```python
from build123d import *

# Parameters (mm, degrees)
F1_DEPTH = 12.7


with BuildPart() as f1:
    # F0 (on Front) → F1 (new body, symmetric)
    with BuildSketch(Plane.XZ):
        with BuildLine():
            Line((46.891703, 59.056909), (0, 59.056909))
            Line((0, 59.056909), (0, 7.407219))
            Line((0, 7.407219), (10.16, 7.407219))
            Line((10.16, 7.407219), (10.16, 46.356909))
            Line((10.16, 46.356909), (34.191703, 46.356909))
            Line((34.191703, 46.356909), (34.191703, -17.143091))
            ThreePointArc((34.191703, -17.143091), (59.591703, -42.543091), (84.991703, -17.143091))
            Line((84.991703, -17.143091), (84.991703, -2.438421))
            Line((84.991703, -2.438421), (72.291703, -2.438421))
            Line((72.291703, -2.438421), (72.291703, -17.143091))
            ThreePointArc((72.291703, -17.143091), (59.591703, -29.843091), (46.891703, -17.143091))
            Line((46.891703, -17.143091), (46.891703, 59.056909))
        make_face()
    extrude(amount=F1_DEPTH, both=True)


solid = f1.part
```
Input: part model. Units: mm. Frame: model coordinates. A direction names the side the tool comes from. Round coordinates to 2 decimals unless told otherwise and drop trailing zeros. Write each loop counter-clockwise with the first axis right and the second up, starting at its lowest first coordinate (ties: lowest second). Pieces come first, ordered by that corner, then holes. Notation, with made-up numbers: (43.25, 46.5) - (49.25, 46.5) arc R26 ccw to (49.25, 61.5) - close; hole circle Ø9 at (87.5, -24.75). An arc over 180 degrees is marked (long way). Write item = value, one per line.
(1) Section query C-C on z = -6.5. Output: boundary loops of the cut face in (x, y).
Geometry check:
outline = (34.19, -12.7) - (46.89, -12.7) - (46.89, 12.7) - (34.19, 12.7) - close; (72.29, -12.7) - (84.99, -12.7) - (84.99, 12.7) - (72.29, 12.7) - close
(2) Material intervals for probe 1 along X at (y, z) = (-10, -3); probe 2 along X at (y, z) = (1.25, 17); probe 3 along X at (y, z) = (10.25, 55.5), sorted ascending.
Geometry check:
probe_1 = 34.19 to 46.89, 72.29 to 84.99
probe_2 = 0 to 10.16, 34.19 to 46.89
probe_3 = 0 to 46.89
(3) Section query A-A on z = 23.5. Output: boundary loops of the cut face in (x, y).
Geometry check:
outline = (0, -12.7) - (10.16, -12.7) - (10.16, 12.7) - (0, 12.7) - close; (34.19, -12.7) - (46.89, -12.7) - (46.89, 12.7) - (34.19, 12.7) - close
(4) Contact query for flat-ended pins moving along their axis: pin 1 Ø7.5 at (y, z) = (4, 35) entering from +X; pin 2 Ø7.5 at (y, z) = (-5.5, -9.5) entering from -X; pin 3 Ø3 at (y, z) = (5.5, 24.5) entering from -X; pin 4 Ø10 at (x, y) = (77.5, 3) entering from +Z. Output: stop coordinate, or through.
Geometry check:
pin_1 = 46.89
pin_2 = 34.19
pin_3 = 0
pin_4 = -2.44
(5) Pull-direction query (X, two-part tool) for faces 4 (the flat face through (39, 12.7, 8)), 5 (the flat face through (22, 0, 46.357)), 6 (the flat face through (0, 0, 34)); classes: +X half, -X half, draft (parallel to the pull), parting line (faces both ways), or undercut.
Geometry check:
face_4 = draft
face_5 = undercut
face_6 = -X half
(6) Section query D-D on x = 59. Output: boundary loops of the cut face in (y, z), then the cut area to 3 significant figures.
Geometry check:
outline = (-12.7, -42.54) - (12.7, -42.54) - (12.7, -29.83) - (-12.7, -29.83) - close
area = 323 mm^2
(7) Section query B-B on y = -10.75. Output: boundary loops of the cut face in (x, z).
Geometry check:
outline = (0, 7.41) - (10.16, 7.41) - (10.16, 46.36) - (34.19, 46.36) - (34.19, -17.14) arc R25.4 ccw to (84.99, -17.14) - (84.99, -2.44) - (72.29, -2.44) - (72.29, -17.14) arc R12.7 cw to (46.89, -17.14) - (46.89, 59.06) - (0, 59.06) - close
(8) Access query for faces 1 (the flat face through (72.292, 0, -10)), 2 (the flat face through (79, 0, -2.438)), 3 (the flat face through (5, 0, 7.407)). Directions: +Z, -Z, +X, -X, +Y, -Y. A direction counts if a zero-diameter tool reaches every point of the face in a straight line with its end or side. Return the directions, or none.
Geometry check:
face_1 = +Z, +Y, -Y
face_2 = +Z, +X, +Y, -Y
face_3 = -Z, -X, +Y, -Y
